Geometry check sheet. Reference: the model listing, model coordinates, mm. A direction names the side the tool comes from. Round coordinates to 2 decimals unless told otherwise and drop trailing zeros. Write each loop counter-clockwise with the first axis right and the second up, starting at its lowest first coordinate (ties: lowest second). Pieces come first, ordered by that corner, then holes. Notation, with made-up numbers: (60, 62) -> (104, 62) arc R20 ccw to (104, 68) -> close; hole circle Ø10 at (10.5, 82). An arc over 180 degrees is marked (long way). Use a Markdown table: item, result.
Solid Edge part; units mm, degrees
sketch "Sketch1" plane through (0, 0, 0) normal (0, 0, 1) x (1, 0, 0)
  line L0 (22.5, -55.25) -> (22.5, 24.75)
  line L1 (-22.5, 24.75) -> (22.5, 24.75)
  line L2 (-22.5, 24.75) -> (-22.5, -55.25)
  line L3 (-22.5, -55.25) -> (22.5, -55.25)
extrude "Protrusion1" add sketch "Sketch1" along normal blind 5
sketch "Sketch2" plane through (0, 55.25, 2.5) normal (0, 1, 0) x (-1, 0, 0)
  line L0 (-20.75, 0) -> (-20.75, 2.5)
  line L1 (-20.75, 2.5) -> (-21.5, 2.5)
  line L2 (-21.5, 2.5) -> (-21.5, -0.5)
  line L3 (-21.5, -0.5) -> (-20, -0.5)
  line L4 (-20, -0.5) -> (-20, 0)
  line L5 (-20, 0) -> (-20.75, 0)
extrude "Cutout1" cut sketch "Sketch2" against normal blind 110.5
mirror "Mirror1" about plane through (0, -55.25, 5) normal (1, 0, 0) of "Cutout1"
sketch "Sketch3" plane through (0, 0, 0) normal (0, 0, -1) x (1, 0, 0)
  line L0 (12.5, 90.25) -> (-22.5, 55.25)
  line L1 (-22.5, 55.25) -> (22.5, 55.25)
  line L2 (22.5, 55.25) -> (22.5, 90.25)
  line L3 (22.5, 90.25) -> (12.5, 90.25)
extrude "Protrusion2" add sketch "Sketch3" against normal blind 5
sketch "Sketch4" plane through (30, -72.75, 2.5) normal (-0.7071, 0.7071, 0) x (0, 0, -1)
  line L0 (-2.5, 24.0416) -> (0.5, 24.0416)
  line L1 (0.5, 24.0416) -> (0.5, 22.2487)
  line L2 (0.5, 22.2487) -> (0, 22.2487)
  line L3 (0, 22.2487) -> (0, 23.5113)
  line L4 (0, 23.5113) -> (-2.5, 23.5113)
  line L5 (-2.5, 23.5113) -> (-2.5, 24.0416)
extrude "Cutout3" cut sketch "Sketch4" along normal blind 48.7806
sketch "Sketch5" plane through (30, -72.75, 2.5) normal (-0.7071, 0.7071, 0) x (0, 0, -1)
  line L0 (-2.5, 23.5113) -> (-2.5, 24.0416)
  line L1 (-2.5, 24.0416) -> (0.5, 24.0416)
  line L2 (0.5, 24.0416) -> (0.5, 22.2487)
  line L3 (0.5, 22.2487) -> (0, 22.2487)
  line L4 (0, 22.2487) -> (0, 23.5113)
  line L5 (0, 23.5113) -> (-2.5, 23.5113)
extrude "Vyříznutí_4" cut sketch "Sketch5" against normal blind 2.7044
sketch "Sketch6" plane through (0.875, -32.75, 5) normal (0, 0, 1) x (0, 1, 0)
  line L0 (-56.5202, -13.1407) -> (-56.5, -21.625)
  line L1 (-57.5, -21.625) -> (-56.5, -21.625)
  line L2 (-57.5, -21.625) -> (-57.5, -15.1605)
  line L3 (-57.5, -15.1605) -> (-57.5, -14.1205)
  line L4 (-57.5, -14.1205) -> (-56.5202, -13.1407)
extrude "Protrusion3" add sketch "Sketch6" along normal blind 13
(1) Release check for a two-part mould opening along X. For faces 6 (the face through (-22, -28, 5)), 7 (the face through (22.5, -33, 2)), 8 (the face through (-20.75, -15, 4)) record: +X half, -X half, draft (parallel to the pull), parting line (faces both ways), or undercut.
A:
| item | result |
|---|---|
| face 6 | draft |
| face 7 | +X half |
| face 8 | undercut |
(2) Section check D-D on y = -20. Record the cut outline in (x, z).
A:
| item | result |
|---|---|
| outline | (-22.5, 0) -> (22.5, 0) -> (22.5, 5) -> (21.5, 5) -> (21.5, 2) -> (20, 2) -> (20, 2.5) -> (20.75, 2.5) -> (20.75, 5) -> (-20.75, 5) -> (-20.75, 2.5) -> (-20, 2.5) -> (-20, 2) -> (-21.5, 2) -> (-21.5, 5) -> (-22.5, 5) -> close |
(3) Thickness scan on line 1 (Z direction, x = -13, y = -13); line 2 (Y direction, x = 5, z = 4); line 3 (X direction, y = -75, z = 3). Record the ranges inside material, lowest first.
A:
| item | result |
|---|---|
| line 1 | z = 0 to 5 |
| line 2 | y = -82.75 to -81.75, -81 to 24.75 |
| line 3 | x = -2.75 to -1.75, -1 to 22.5 |
(4) Section check A-A on y = -56.5. Record the cut outline in (x, z), plus the area to 3 significant figures.
A:
| item | result |
|---|---|
| outline | (-21.25, 0) -> (22.5, 0) -> (22.5, 5) -> (-19.5, 5) -> (-19.5, 2.5) -> (-17.71, 2.5) -> (-17.71, 2) -> (-20.25, 2) -> (-20.25, 5) -> (-21.25, 5) -> close |
| area | 216 mm2 |
(5) Section check B-B on x = 4. Record the cut outline in (y, z).
A:
| item | result |
|---|---|
| outline | (-81.75, 0) -> (24.75, 0) -> (24.75, 5) -> (-80, 5) -> (-80, 2.5) -> (-78.21, 2.5) -> (-78.21, 2) -> (-80.75, 2) -> (-80.75, 5) -> (-81.75, 5) -> close |
(6) Access from +Z, -Z, +X, -X, +Y, -Y to the whole of each face (thin tool, end or side, straight path). Record for faces 1 (the face through (-2.234, -71.98, 2.246)), 2 (the face through (-3, -73, 4)), 3 (the face through (1, -32, 5)), 4 (the face through (21.5, -15, 4)), 5 (the face through (0, 24.75, 2)).
A:
| item | result |
|---|---|
| face 1 | none |
| face 2 | +Z |
| face 3 | +Z, +X, -X, +Y |
| face 4 | +Z, +Y |
| face 5 | +Z, -Z, +X, -X, +Y |
(7) Section check C-C on z = 8.5. Record the cut outline in (x, y).
A:
| item | result |
|---|---|
| outline | (14.02, -89.27) -> (15, -90.25) -> (22.5, -90.25) -> (22.5, -89.25) -> close |
(8) Gauge pin test, flat end, axial feed: pin 1 Ø21.5 at (x, y) = (6, -10) entering from +Z. Record the tip position at first contact, or that the pin passes through.
A:
| item | result |
|---|---|
| pin 1 | stops at z = 5 |
